Here's how the part is built. I have some questions about the finished solid (model axes, mm). Face numbers are marked on the shaded views. A direction names the side the tool comes from. Round coordinates to 2 decimals unless told otherwise and drop trailing zeros. Order: outer loops, then holes, each group sorted by start corner. A loop starts at its lowest first (then second) coordinate and runs counter-clockwise, first axis right, second up. Notation, with made-up numbers: M 48.25,86.5 L 75.25,86.5 A27 cw 75.25,121.5 Z; hole C -40,15.25 d9. An arc over 180 degrees is marked long. Write item = value, one per line. Start each with the question number.
Item 1: I want a section at B-B, the plane z = -2.5. List the corners of the cut face in (x, y) for me, plus the area to 3 significant figures.
Item 2: I want a section at C-C, the plane y = 4.5. List the corners of the cut face in (x, z) for me.
Item 3: I want a section at D-D, the plane x = -2. List the corners of the cut face in (y, z) for me.
Item 4: I'm going to push flat-ended pins straight in: P1, Ø3, axis at y = 31, z = 0.5, coming from the -X side; P2, Ø6, axis at x = 2.5, z = -2.5, coming from the -Y side; P3, Ø1, axis at y = 20, z = -2, coming from the +X side; P4, Ø2, axis at y = 52.5, z = -4, coming from the +X side. Where does each tip first touch, or does it pass through?
Item 5: I want a section at A-A, the plane y = 16.5. List the corners of the cut face in (x, z) for me, plus the area to 3 significant figures.
Item 6: Please list where these lines run through material, in increasing order: L1, parallel to Z at x = 0, y = 5; L2, parallel to Y at x = -4.25, z = -1; L3, parallel to X at y = 11, z = -0.5.
Item 7: For the marked faces 1, 2 and 3, which set-ups out of +Z, -Z, +X, -X, +Y, -Y let a thin tool reach every point of the face, with its end or its side?
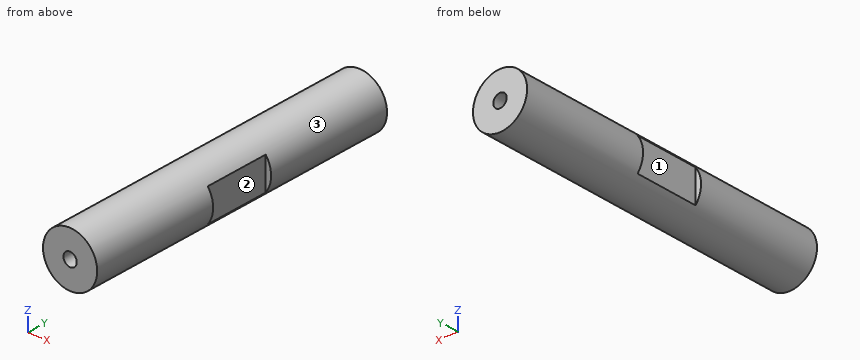
Autodesk Inventor part; units mm, degrees
ref_plane "YZ Plane" through (0, 0, 0) normal (1, 0, 0) x (0, 1, 0)
ref_plane "XZ Plane" through (0, 0, 0) normal (0, 1, 0) x (-1, 0, 0)
ref_plane "XY Plane" through (0, 0, 0) normal (0, 0, 1) x (1, 0, 0)
sketch "Sketch1" plane through (0, 0, 0) normal (0, 1, 0) x (-1, 0, 0)
  circle A0 centre (0, 0) radius 5
  dimension "d0" = 10
extrude "Extrusion1" add sketch "Sketch1" along normal blind 60
sketch "Sketch2" plane through (0, 60, 0) normal (0, 1, 0) x (1, 0, 0)
  point P0 (0, 0)
  point P1 (0, 0)
hole "Hole1" at (0, 60, 0) direction (0, -1, 0) diameter 2.459 depth 12 tip angle 118
sketch "Sketch3" plane through (0, 0, 0) normal (0, -1, 0) x (1, 0, 0)
  circle A0 centre (0, 0) radius 1.2295
hole "Hole2" at (0, 0, 0) direction (0, 1, 0) diameter 2.459 depth 12 tip angle 118
sketch "Sketch4" plane through (0, 0, 0) normal (0, 0, 1) x (1, 0, 0)
  line L0 (-5, 0) -> (-5, 60)
  line L1 (5, 0) -> (5, 60)
  line L2 (-5, 0) -> (5, 0)
  line L3 (5, 60) -> (-5, 60)
  line L4 (-5, 24) -> (-4, 24)
  line L5 (-4, 24) -> (-4, 36)
  line L6 (-4, 36) -> (-5, 36)
  line L7 (5, 24) -> (4, 24)
  line L8 (4, 24) -> (4, 36)
  line L9 (4, 36) -> (5, 36)
  line L10 (-5, 36) -> (-15, 36)
  line L11 (-15, 36) -> (-15, 24)
  line L12 (-15, 24) -> (-5, 24)
  line L13 (5, 36) -> (15, 36)
  line L14 (15, 36) -> (15, 24)
  line L15 (15, 24) -> (5, 24)
  point P0 (0, 0)
  point P1 (-4.5, 24)
  dimension "d17" = 60
  dimension "d18" = 12
  dimension "d19" = 24
  dimension "d20" = 1
  dimension "d21" = 1
  dimension "d22" = 10
  dimension "d23" = 10
extrude "Extrusion2" cut sketch "Sketch4" along normal mid plane 10 contours L12 L11 L10 L0 | L0 L6 L5 L4 | L7 L8 L9 L1 | L1 L13 L14 L15
equation "\"d21\" = d20"
equation "\"d23\" = d22"
properties part number "Post-2023-1" material "Copper"
Filled in:
q1.outline = M -4.33,0 L 4.33,0 L 4.33,24 L 4,24 L 4,36 L 4.33,36 L 4.33,60 L -4.33,60 L -4.33,36 L -4,36 L -4,24 L -4.33,24 Z
q1.area = 512 mm^2
q2.outline = C 0,0 d10; hole C 0,0 d2.46
q3.outline = M 0,-4.58 L 60,-4.58 L 60,4.58 L 0,4.58 Z
q4.P1 = -4
q4.P2 = 0
q4.P3 = 4.77
q4.P4 = 4
q5.outline = C 0,0 d10
q5.area = 78.5 mm^2
q6.L1 = -5 to -1.23, 1.23 to 5
q6.L2 = 0 to 24, 36 to 60
q6.L3 = -4.97 to -1.12, 1.12 to 4.97
q7.face_1 = +Z, -Z, -X
q7.face_2 = +Z, -Z, +X
q7.face_3 = +Y, -Y
